Autodesk Fusion 360 part; units mm, degrees
sketch "Sketch1" plane through (0, 0, 0) normal (0, 0, 1) x (1, 0, 0)
  line L0 (17, 4) -> (-17, 4)
  line L1 (-17, 4) -> (-17, -4)
  line L2 (-17, -4) -> (17, -4)
  line L3 (17, -4) -> (17, 4)
  line L4 (17, 4) -> (-17, -4) construction
  line L5 (-17, 4) -> (17, -4) construction
  line L6 (0, 0) -> (14, 0) construction
  circle A0 centre (14, 0) radius 1.5
  line L7 (0, 0) -> (0, 4) construction
  circle A1 centre (-14, 0) radius 1.5
  line L8 (11, 2) -> (-11, 2)
  line L9 (-11, 2) -> (-11, -2)
  line L10 (-11, -2) -> (11, -2)
  line L11 (11, -2) -> (11, 2)
  line L12 (11, 2) -> (-11, -2) construction
  line L13 (-11, 2) -> (11, -2) construction
  line L14 (-11, -4) -> (11, -4)
  line L15 (11, -4) -> (11, 4)
  line L16 (11, 4) -> (-11, 4)
  line L17 (-11, 4) -> (-11, -4)
  line L18 (-11, -4) -> (11, 4) construction
  line L19 (11, -4) -> (-11, 4) construction
  dimension "d44" = 34
  dimension "d45" = 14
  dimension "d46" = 3
  dimension "d47" = 3
  dimension "d48" = 2
  dimension "d49" = 8
  dimension "d54" = 22
extrude "Extrude4" add sketch "Sketch1" against normal blind 12 contours L0 L2 L3 L11 L15 | L0 L8 L15 L16 L17 | L0 L1 L2 L9 L17 | L2 L10 L14 L15 L17
fillet "Fillet5" radius 2 8 edges at (-17, -4, -6) (17, -4, -6) (17, 4, -6) (-17, 4, -6) (-11, 2, -6) (-11, -2, -6) (11, -2, -6) (11, 2, -6)
thread "Thread4"
extrude "Extrude5" cut sketch "Sketch1" against normal blind 2 contours L0 L8 L15 L16 L17 | L8 L9 L10 L11 L15 L17 | L2 L10 L14 L15 L17
fillet "Fillet6" radius 1 2 edges at (-11, 0, 0) (11, 0, 0)
equation "d1 = ( 47 / 2 ) * 1 mm"
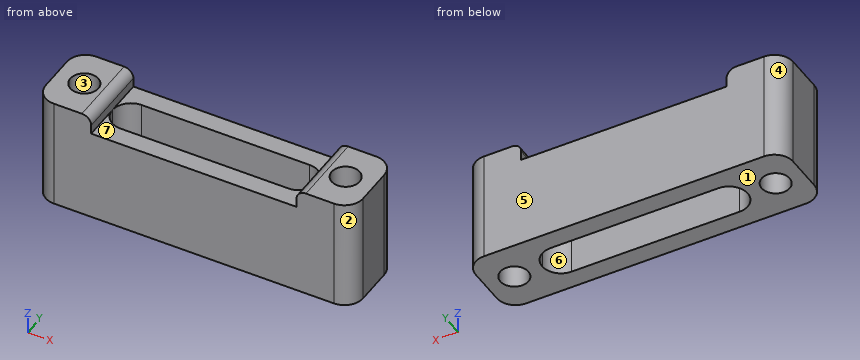
Geometry check sheet. Reference: the model listing, model coordinates, mm. Face numbers are marked on the shaded views. A direction names the side the tool comes from. Coordinates: 2 decimals unless noted, no trailing zeros. Order: outer loops, then holes, each group sorted by start corner. A loop starts at its lowest first (then second) coordinate and runs counter-clockwise, first axis right, second up. Notation, with made-up numbers: M -27,89.5 L 24,89.5 A22 ccw 24,103.5 Z; hole C -19,75 d9. An arc over 180 degrees is marked long. One line per question, with ' | ' between items. Start each with the question number.
Item 1: Cross-section at C-C on x = -14. Enter the section's corners in (y, z).
Item 2: Set-up check for the marked faces 5, 6 and 7: record each of +Z, -Z, +X, -X, +Y, -Y from which the full face is reachable in a straight line by a thin tool's end or side.
Item 3: Cross-section at A-A on x = 2. Enter the section's corners in (y, z).
Item 4: Draft check along X on the marked faces 1, 2, 3 and 4. Enter one of: pulls with the +X half, pulls with the -X half, needs draft (parallel to the pull), parting line crosses it, or undercut.
Item 5: Material ranges on L1, parallel to Y at x = 14, z = -3.75; L2, parallel to Y at x = -9, z = -9; L3, parallel to X at y = -0.75, z = -8.25, recorded low to high. Write a range as [from, to].
Item 6: Cross-section at B-B on z = -4. State how many separate pieces and enclosed holes the cut face has, then the cut area to 3 significant figures.
Item 7: Cross-section at D-D on y = -0.5. Enter the section's corners in (x, z), then the cut area to 3 significant figures.
Item 8: Gauge pin test, flat ends, axial feed: pin 1 (1.2 mm diameter, centred on x = -3.5, y = -2, fed in from +Z); pin 2 (2.5 mm diameter, centred on x = 14, y = 0, fed in from +Z). Record the tip position at first contact, or that the pin passes through.
Findings:
1) outline: M -4,-12 L -1.5,-12 L -1.5,0 L -4,0 Z; M 1.5,-12 L 4,-12 L 4,0 L 1.5,0 Z
2) face 5: +Z, -Z, +X, -X, +Y | face 6: +Z, -Z | face 7: +Z, +Y, -Y
3) outline: M -4,-12 L -2,-12 L -2,-2 L -4,-2 Z; M 2,-12 L 4,-12 L 4,-2 L 2,-2 Z
4) face 1: needs draft | face 2: pulls with the +X half | face 3: undercut | face 4: pulls with the -X half
5) L1: y = [-4, -1.5], [1.5, 4] | L2: y = [-4, -2], [2, 4] | L3: x = [-17, -15.3], [-12.7, -10.85], [10.85, 12.7], [15.3, 17]
6) separate pieces: 1 | enclosed holes: 3 | area: 170 mm²
7) outline: M -17,-12 L -15.41,-12 L -15.41,0 L -17,0 Z; M -12.59,-12 L -10.94,-12 L -10.94,-2 L -11,-2 L -11,-1 A1 ccw -12,0 L -12.59,0 Z; M 10.94,-12 L 12.59,-12 L 12.59,0 L 12,0 A1 ccw 11,-1 L 11,-2 L 10.94,-2 Z; M 15.41,-12 L 17,-12 L 17,0 L 15.41,0 Z | area: 77.0 mm²
8) pin 1: stops at z = -2 | pin 2: passes through
